Read the model definition and answer for the solid it produces. Units are mm, in the model's axes. A direction names the side the tool comes from. Round coordinates to 2 decimals unless told otherwise and drop trailing zeros. Order: outer loops, then holes, each group sorted by start corner. A loop starts at its lowest first (then second) coordinate and runs counter-clockwise, first axis right, second up. Notation, with made-up numbers: (33, 35) - (48, 35) arc R12 ccw to (48, 53) - close; hole circle Ø4 at (75.25, -25). An arc over 180 degrees is marked (long way). One line per question, with ' | ' between items. Start each with the question number.
1) The part is cut by section B-B, the plane x = 0. Give the vertices of the cut face in (y, z), plus the area to 3 significant figures.
2) The part is cut by section D-D, the plane z = 46.5. Give the vertices of the cut face in (x, y).
3) The mould has two halves that part along Z. Classify faces 5 (the cylindrical face through (33.37, -1.01, 11.81)), 6 (the flat face through (-13.87, -0.99, 4.8)), 7 (the cylindrical face through (35.07, -0.99, 7.92)): pulls with the +Z half, pulls with the -Z half, needs draft (parallel to the pull), parting line crosses it, or undercut.
4) For faces 1 (the flat face through (19.93, -0.986, 9.262)), 2 (the cylindrical face through (-0.78, -0.99, 29.31)), 3 (the flat face through (-4.327, -1, 45)), 4 (the flat face through (5.846, -1, 46)), determine the directions among +Z, -Z, +X, -X, +Y, -Y from which every point of the face is accessible in a straight line to the end or side of a thin tool.
5) Flat-ended cylindrical pins translate along their axes: pin 1 (4 mm diameter, centred on x = -21.05, z = 5.16, fed in from -Y); pin 2 (0.6 mm diameter, centred on y = -1, z = 48, fed in from +X). Find the tip coordinate at first contact, or state that the pin passes through.
6) Straight lines are drawn through the part: line 1 (Z direction, x = 0, y = -0.5); line 2 (X direction, y = -0.85, z = 44); line 3 (X direction, y = -0.2, z = 24). For each, find the intervals that lie inside material, in ascending order. Write a range as from..to.
7) The part is cut by section A-A, the plane z = 12. Give the vertices of the cut face in (x, y), plus the area to 3 significant figures.
8) The part is cut by section C-C, the plane y = -0.85. Give the vertices of the cut face in (x, z), plus the area to 3 significant figures.
from build123d import *

# Parameters (mm, degrees)
F0_R     = 6
F3_DEPTH = 2
F4_R     = 2.937220037
F4_R_2   = 2.9600798579
F4_R_3   = 3.1369542822
F5_DEPTH = 25
F6_R     = 3.870285665
F6_R_2   = 3.4699614842
F7_DEPTH = 3


# Not quite as in the source:
# - the program builds the solid bodies; features that only make, move or delete a surface that nothing else refers to are left out


with BuildPart() as f3:
    # F0 (on Front) → F3 (new body)
    with BuildSketch(Plane.XZ):
        with BuildLine():
            ThreePointArc((19.6806687258, 19.8017779916), (19.9200072103, 21.5744676649), (20, 23.3614519238))
            ThreePointArc((20, 23.3614519238), (16.0767393697, 35.2584452936), (5.8461548761, 42.4879380926))
            ThreePointArc((5.8461548761, 42.4879380926), (0.7853649586, 43.3460260219), (-4.327156771, 42.8877345777))
            ThreePointArc((-4.327156771, 42.8877345777), (-17.6128349493, 32.8371073128), (-18.6785365647, 16.2121672183))
            ThreePointArc((-18.6785365647, 16.2121672183), (-15.8565738824, 11.1725608869), (-11.7121291204, 7.1495417506))
            ThreePointArc((-11.7121291204, 7.1495417506), (2.6572751847, 3.5387657135), (15.5683835849, 10.8065551679))
            ThreePointArc((15.5683835849, 10.8065551679), (18.189349373, 15.0459501719), (19.6806687258, 19.8017779916))
        make_face()
        with Locations((0, 23.3614519238)):
            Circle(F0_R, mode=Mode.SUBTRACT)
        with BuildLine():
            ThreePointArc((-4.327156771, 42.8877345777), (0.7853649586, 43.3460260219), (5.8461548761, 42.4879380926))
            Line((5.8461548761, 42.4879380926), (5.8461548761, 50.2402076719))
            ThreePointArc((5.8461548761, 50.2402076719), (-1.3985114704, 58.4135951865), (-4.327156771, 47.891594871))
            Line((-4.327156771, 47.891594871), (-4.327156771, 42.8877345777))
        make_face()
        with BuildLine():
            Line((28.5979291758, 16.5996841985), (19.6806687258, 19.8017779916))
            ThreePointArc((19.6806687258, 19.8017779916), (18.189349373, 15.0459501719), (15.5683835849, 10.8065551679))
            Line((15.5683835849, 10.8065551679), (24.4160998295, 7.6740266873))
            ThreePointArc((24.4160998295, 7.6740266873), (35.1512386763, 8.0868826224), (28.5979291758, 16.5996841985))
        make_face()
        with BuildLine():
            ThreePointArc((-11.7121291204, 7.1495417506), (-15.8565738824, 11.1725608869), (-18.6785365647, 16.2121672183))
            Line((-18.6785365647, 16.2121672183), (-25.2698698947, 9.0414457989))
            ThreePointArc((-25.2698698947, 9.0414457989), (-24.3393468403, 0.4704595262), (-15.965672237, 2.5221058119))
            Line((-15.965672237, 2.5221058119), (-11.7121291204, 7.1495417506))
        make_face()
    extrude(amount=F3_DEPTH)

    # F4 (on Front) → F5 (cut)
    with BuildSketch(Plane.XZ):
        with Locations((0, 53.6376424134)):
            Circle(F4_R)
        with Locations((29.5011680573, 10.3136152029)):
            Circle(F4_R_2)
        with Locations((-20.7987613976, 4.8063262366)):
            Circle(F4_R_3)
    extrude(amount=-F5_DEPTH, mode=Mode.SUBTRACT)

    # F6 (on face) → F7 (cut)
    with BuildSketch(Plane.XZ.offset(2)):
        with Locations((29.6770948917, 10.6516163796)):
            Circle(F6_R)
        with Locations((-21.0510119796, 5.1634679548)):
            Circle(F6_R_2)
    extrude(amount=-F7_DEPTH, mode=Mode.SUBTRACT)


solid = f3.part
Values:
1) outline: (-2, 3.36) - (0, 3.36) - (0, 17.36) - (-2, 17.36) - close; (-2, 29.36) - (0, 29.36) - (0, 58.57) - (-2, 58.57) - close | area: 86.4 mm^2
2) outline: (-4.33, -2) - (5.85, -2) - (5.85, 0) - (-4.33, 0) - close
3) face 5: undercut | face 6: pulls with the -Z half | face 7: parting line crosses it
4) face 1: -Z, +Y, -Y | face 2: +Y, -Y | face 3: -X, +Y, -Y | face 4: +X, +Y, -Y
5) pin 1: passes through | pin 2: stops at x = 5.85
6) line 1: z = 3.36..17.36, 29.36..58.57 | line 2: x = -4.33..5.85 | line 3: x = -19.99..-5.97, 5.97..19.99
7) outline: (-22.55, -2) - (26.05, -2) - (26.05, 0) - (-22.55, 0) - close; (33.3, -2) - (35.57, -2) - (35.57, 0) - (33.3, 0) - close | area: 102 mm^2
8) outline: (-25.27, 9.04) arc R5.73 ccw (long way) to (-15.97, 2.52) - (-11.71, 7.15) arc R20 ccw to (15.57, 10.81) - (24.42, 7.67) arc R6.05 ccw (long way) to (28.6, 16.6) - (19.68, 19.8) arc R20 ccw to (5.85, 42.49) - (5.85, 50.24) arc R6.22 ccw (long way) to (-4.33, 47.89) - (-4.33, 42.89) arc R20 ccw to (-18.68, 16.21) - close; hole circle Ø6.94 at (-21.05, 5.16); hole circle Ø12 at (0, 23.36); hole circle Ø7.74 at (29.68, 10.65) | area: 1,550 mm^2
